Check sheet for the drawn part. Datum: minimum x, y, z corner. Units: mm. A direction names the side the tool comes from. Round coordinates to 2 decimals unless told otherwise and drop trailing zeros. Write each loop counter-clockwise with the first axis right and the second up, starting at its lowest first coordinate (ties: lowest second). Pieces come first, ordered by that corner, then holes.
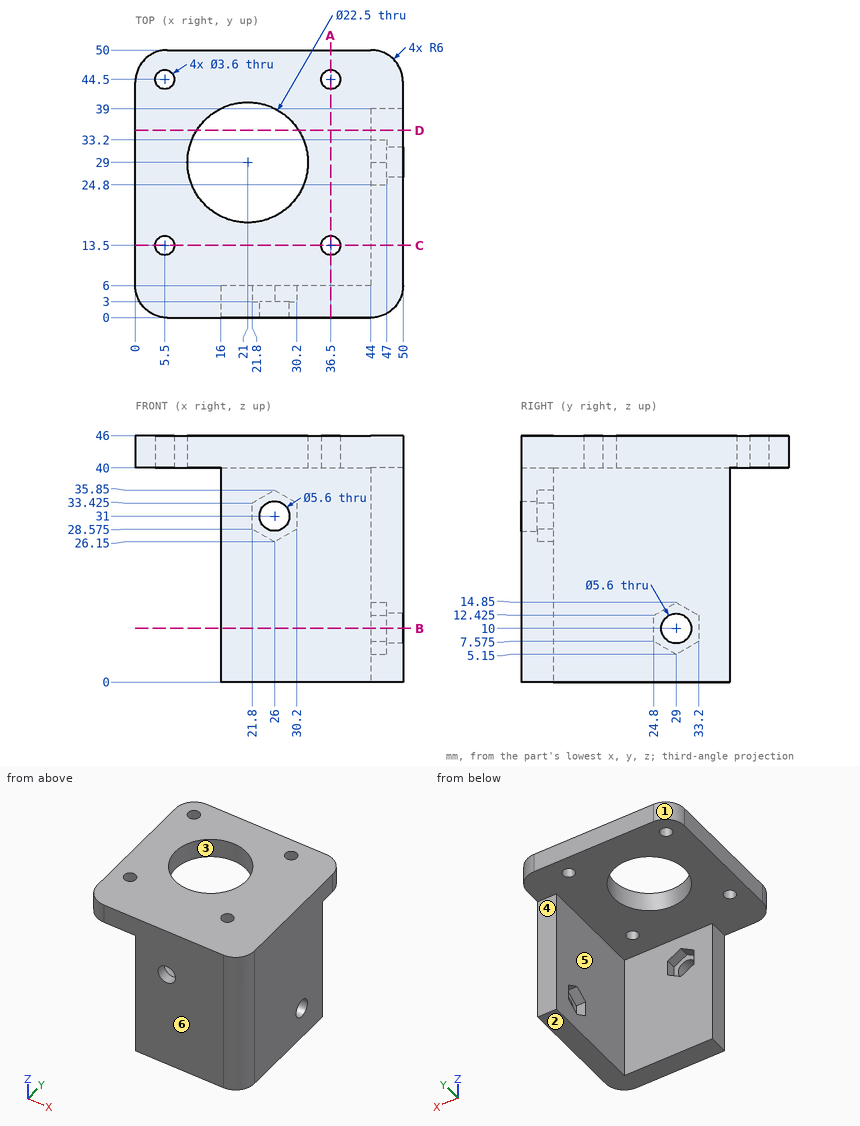
1. Set-up check for the marked faces 4, 5 and 6: record each of +Z, -Z, +X, -X, +Y, -Y from which the full face is reachable in a straight line by a thin tool's end or side.
2. Scan lines: line 1 along Z through (x, y) = (48, 29); line 2 along Y through (x, z) = (5, 43); line 3 along Y through (x, z) = (21, 43.7). Record each from-to range of solid material in increasing order.
3. Sectioned sample at B-B, the plane z = 10. Enter the section's corners in (x, y).
4. Go/stop test with flat-tipped pins: pin 1 (9 mm diameter, centred on y = 28, z = 8.5, fed in from -X); pin 2 (2.5 mm diameter, centred on x = 25.5, z = 29.5, fed in from +Y); pin 3 (22.5 mm diameter, centred on x = 25, z = 15, fed in from +Y); pin 4 (10 mm diameter, centred on y = 30.5, z = 39.5, fed in from -X). Record where each tip stops, or that it passes through.
5. Sectioned sample at C-C, the plane y = 13.5. Enter the section's corners in (x, z).
6. Release check for a two-part mould opening along X. For the marked faces 1, 2 and 3 record: released by +X, released by -X, zero draft, split by the parting line, or undercut.
7. Sectioned sample at A-A, the plane x = 36.5. Enter the section's corners in (y, z), plus the area to 3 significant figures.
8. Sectioned sample at D-D, the plane y = 35. Enter the section's corners in (x, z).
Computed values:
1. face 4: -Z, +X, -X, +Y
1. face 5: -Z, -X, +Y
1. face 6: +Z, -Z, +X, -X, -Y
2. line 1: z = 0 to 7.2, 12.8 to 46
2. line 2: y = 0.08 to 11.77, 15.23 to 42.77, 46.23 to 49.92
2. line 3: y = 0 to 17.75, 40.25 to 50
3. outline: (16, 0) - (44, 0) arc R6 ccw to (50, 6) - (50, 26.2) - (47, 26.2) - (47, 24.8) - (44, 24.8) - (44, 6) - (16, 6) - close; (44, 33.2) - (47, 33.2) - (47, 31.8) - (50, 31.8) - (50, 39) - (44, 39) - close
4. pin 1: stops at x = 44
4. pin 2: stops at y = 3
4. pin 3: stops at y = 6
4. pin 4: stops at x = 0
5. outline: (0, 40) - (3.7, 40) - (3.7, 46) - (0, 46) - close; (7.3, 40) - (34.7, 40) - (34.7, 46) - (7.3, 46) - close; (38.3, 40) - (44, 40) - (44, 0) - (50, 0) - (50, 46) - (38.3, 46) - close
6. face 1: released by -X
6. face 2: zero draft
6. face 3: undercut
7. outline: (0, 0) - (6, 0) - (6, 40) - (11.7, 40) - (11.7, 46) - (0, 46) - close; (15.3, 40) - (42.7, 40) - (42.7, 46) - (15.3, 46) - close; (46.3, 40) - (50, 40) - (50, 46) - (46.3, 46) - close
7. area: 497 mm2
8. outline: (0, 40) - (11.48, 40) - (11.48, 46) - (0, 46) - close; (30.52, 40) - (44, 40) - (44, 0) - (50, 0) - (50, 46) - (30.52, 46) - close
